Study the drawing (mm; zero at the part's minimum x, y, z) and answer. A direction names the side the tool comes from. Coordinates: 2 decimals unless noted, no trailing zeros. Order: outer loops, then holes, each group sorted by start corner. A loop starts at its lowest first (then second) coordinate and runs counter-clockwise, first axis right, second up. Notation, with made-up numbers: M -13,35.5 L -5,35.5 A11 cw -5,55.5 Z; hole C 63.5,88.5 d1. An arc over 180 degrees is marked long. Use a Markdown table: item, result. Add a question column.
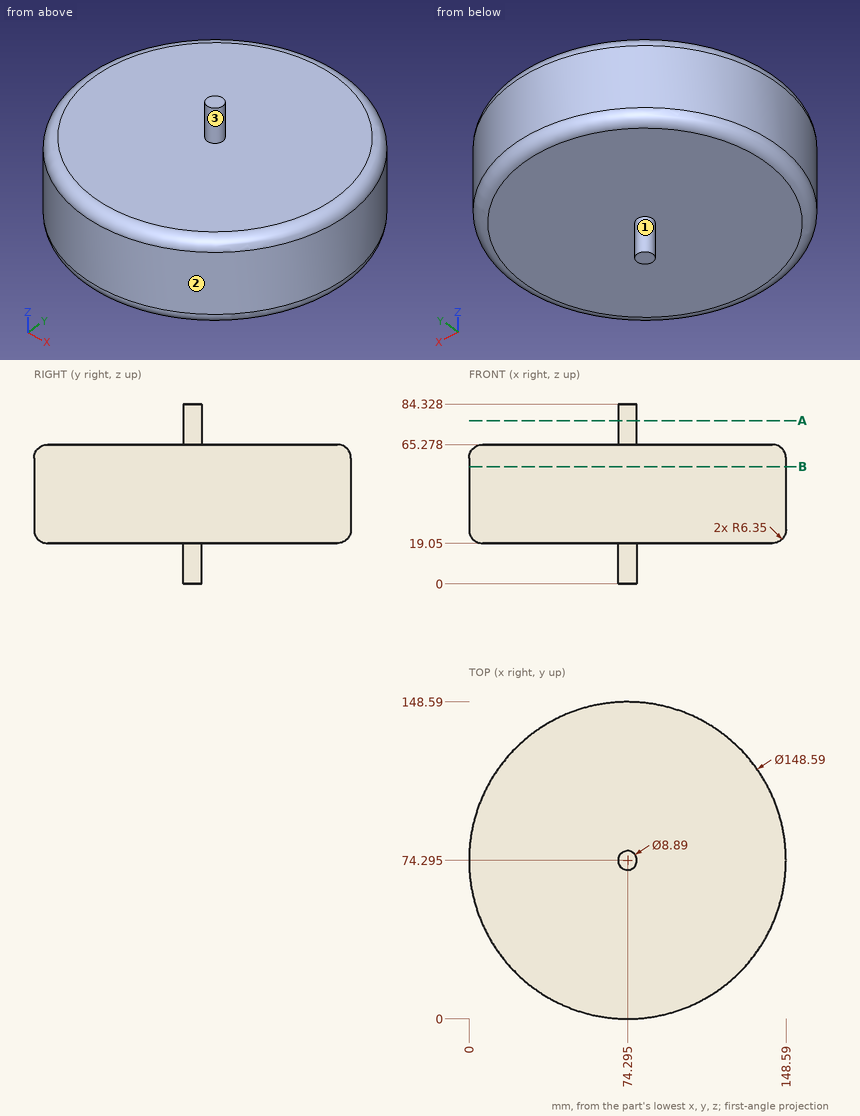
(1) Given P1, Ø3, axis at x = 61, z = 31.5, coming from the -Y side; P2, Ø5, axis at y = 105, z = 31, coming from the +X side; P3, Ø3, axis at y = 89, z = 27.5, coming from the -X side, each flat-ended and moving along its own axis, determine where each tip first touches the part or whether it passes through.
(2) A cutting plane is placed at A-A on z = 76.5. Write down the section's boundary in (x, y) (3 decimals).
(3) Which of the six approach directions +Z, -Z, +X, -X, +Y, -Y give full straight-line access (tool end or side, diameter ignored) to the marked faces 1, 2 and 3?
(4) Straight lines are drawn through the part: line 1 (Z direction, x = 128, y = 52); line 2 (X direction, y = 42, z = 54); line 3 (X direction, y = 99.5, z = 34). For each, find the intervals that lie inside material, in ascending order.
(5) A cutting plane is placed at B-B on z = 55. Write down the section's boundary in (x, y) (3 decimals).
From the geometry:
| question | item | result |
|---|---|---|
| 1 | P1 | stops at y = 0.94 |
| 1 | P2 | stops at x = 143.03 |
| 1 | P3 | stops at x = 1.18 |
| 2 | outline | C 74.295,74.295 d8.89 |
| 3 | face 1 | -Z |
| 3 | face 2 | +Z, -Z |
| 3 | face 3 | +Z |
| 4 | line 1 | z = 19.05 to 65.28 |
| 4 | line 2 | x = 7.39 to 141.2 |
| 4 | line 3 | x = 4.41 to 144.18 |
| 5 | outline | C 74.295,74.295 d148.59 |
